The listing builds one solid part. Answer for the finished solid, in the listing's coordinates (mm). A direction names the side the tool comes from. Give positions to 0.01 mm unless a question says otherwise; leave off trailing zeros. Write each loop counter-clockwise with the first axis right and the second up, starting at its lowest first coordinate (ties: lowest second). Pieces come first, ordered by that corner, then holes. Notation, with made-up numbers: (73.5, 63) - (126.5, 63) arc R11 ccw to (126.5, 67) - close; hole circle Ø11 at (30, 12). An arc over 180 degrees is marked (long way). Answer as CSV lines item,"result". Start each with the question number.
(1) Find section D-D (y = -1). Write down the section's boundary in (x, z).
(2) Find section B-B (x = 47.5). Write down the section's boundary in (y, z), then the cut area to 3 significant figures.
(3) Find section A-A (y = -6). Write down the section's boundary in (x, z), then the cut area to 3 significant figures.
(4) For faces 4 (the face through (52.76, -1.47, 11.07)), 5 (the face through (-39, 7.5, 7)), 6 (the face through (-35.65, 6, 7)), 7 (the face through (16, -5, 0)), 8 (the face through (49, -1, 13.1)), determine the directions among +Z, -Z, +X, -X, +Y, -Y from which every point of the face is accessible in a straight line to the end or side of a thin tool.
(5) Straight lines are drawn through the part: probe 1 along Z at (x, y) = (52.6, -1); probe 2 along X at (y, z) = (3.25, 2.25); probe 3 along X at (y, z) = (-7, 11.5). For each, find the intervals that lie inside material, in ascending order.
(6) Find section C-C (z = 7.5). Write down the section's boundary in (x, y), then the cut area to 3 significant figures.
(7) This flat-tipped pin is pushed along its axis until it touches: pin 1 Ø8 at (x, z) = (28.5, 2.5) entering from +Y. Where does it stop, or does it pass through?
(8) For a pull along Y with two mould halves and no side action, classify faces 1 (the face through (44, 7.5, 7)), 2 (the face through (5, -9.5, 7)), 3 (the face through (49, -1, 1.9)) as pulls with the +Y half, pulls with the -Y half, needs draft (parallel to the pull), parting line crosses it, or undercut.
from build123d import *

# Parameters (mm, degrees)
F1_DEPTH = 15
F2_W     = 13
F2_H     = 11.2
F3_DEPTH = 6
F4_W     = 17
F4_H     = 15
F5_DEPTH = 1.2
F6_R     = 3.6
F7_DEPTH = 2


with BuildPart() as f1:
    # F0 (on Top) → F1 (new body)
    with BuildSketch(Plane.XY):
        with BuildLine():
            ThreePointArc((40.15, 0), (38.831981, -3.181981), (35.65, -4.5))
            Line((35.65, -4.5), (-35.65, -4.5))
            ThreePointArc((-35.65, -4.5), (-38.831981, -3.181981), (-40.15, 0))
            ThreePointArc((-40.15, 0), (-38.831981, 3.181981), (-35.65, 4.5))
            Line((-35.65, 4.5), (-35.65, 7.5))
            Line((-35.65, 7.5), (-42.15, 7.5))
            Line((-42.15, 7.5), (-42.15, -9.5))
            Line((-42.15, -9.5), (52.15, -9.5))
            Line((52.15, -9.5), (52.15, 7.5))
            Line((52.15, 7.5), (35.65, 7.5))
            Line((35.65, 7.5), (35.65, 4.5))
            ThreePointArc((35.65, 4.5), (38.831981, 3.181981), (40.15, 0))
        make_face()
    extrude(amount=F1_DEPTH)

    # F2 (on face) → F3 (cut)
    with BuildSketch(Plane.YZ.offset(52.15)):
        with Locations((-1, 7.5)):
            Rectangle(F2_W, F2_H)
    extrude(amount=-F3_DEPTH, mode=Mode.SUBTRACT)

    # F4 (on face) → F5 (join)
    with BuildSketch(Plane.YZ.offset(52.15)):
        with Locations((-1, 7.5)):
            Rectangle(F4_W, F4_H)
    extrude(amount=F5_DEPTH)

    # F6 (on face) → F7 (cut)
    with BuildSketch(Plane.YZ.offset(53.35)):
        with Locations((-1, 7.5)):
            Circle(F6_R)
    extrude(amount=-F7_DEPTH, mode=Mode.SUBTRACT)


solid = f1.part
Result set:
1,outline,"(-42.15, 0) - (-40.04, 0) - (-40.04, 15) - (-42.15, 15) - close; (40.04, 0) - (53.35, 0) - (53.35, 3.9) - (52.15, 3.9) - (52.15, 1.9) - (46.15, 1.9) - (46.15, 13.1) - (52.15, 13.1) - (52.15, 11.1) - (53.35, 11.1) - (53.35, 15) - (40.04, 15) - close"
2,outline,"(-9.5, 0) - (7.5, 0) - (7.5, 15) - (-9.5, 15) - close; hole (-7.5, 1.9) - (5.5, 1.9) - (5.5, 13.1) - (-7.5, 13.1) - close"
2,area,"109 mm^2"
3,outline,"(-42.15, 0) - (53.35, 0) - (53.35, 15) - (-42.15, 15) - close; hole (46.15, 1.9) - (52.15, 1.9) - (52.15, 13.1) - (46.15, 13.1) - close"
3,area,"1,370 mm^2"
4,face 4,"+X"
4,face 5,"+Z, -Z, +X, -X, +Y"
4,face 6,"+Z, -Z, +Y"
4,face 7,"-Z, +X, -X, +Y, -Y"
4,face 8,"none"
5,probe 1,"0 to 3.9, 11.1 to 15"
5,probe 2,"-42.15 to -38.76, 38.76 to 46.15, 52.15 to 53.35"
5,probe 3,"-42.15 to 46.15, 52.15 to 53.35"
6,outline,"(-42.15, -9.5) - (53.35, -9.5) - (53.35, -4.6) - (52.15, -4.6) - (52.15, -7.5) - (46.15, -7.5) - (46.15, 5.5) - (52.15, 5.5) - (52.15, 2.6) - (53.35, 2.6) - (53.35, 7.5) - (35.65, 7.5) - (35.65, 4.5) arc R4.5 cw to (40.15, 0) arc R4.5 cw to (35.65, -4.5) - (-35.65, -4.5) arc R4.5 cw to (-40.15, 0) arc R4.5 cw to (-35.65, 4.5) - (-35.65, 7.5) - (-42.15, 7.5) - close"
6,area,"618 mm^2"
7,pin 1,"y = -4.5"
8,face 1,"pulls with the +Y half"
8,face 2,"pulls with the -Y half"
8,face 3,"undercut"
